from build123d import *

# Parameters (mm, degrees)
SKETCH_1_W               = 65
SKETCH_1_H               = 70
EXTRUDE_1_DEPTH          = 25
SKETCH_2_R               = 15.75
CUT_EXTRUDE_1_DEPTH      = 26
SKETCH_4_R               = 3
CUT_EXTRUDE_2_DEPTH      = 40
PATTERN_CIRCULAR_1_COUNT = 4
CUT_EXTRUDE_3_DEPTH      = 26
CUT_EXTRUDE_START        = -26
CUT_EXTRUDE_5_DEPTH      = 46
SKETCH_8_R               = 1.25
SKETCH_8_R_2             = 1.5
CUT_EXTRUDE_6_DEPTH      = 10
SKETCH_9_W               = 81.802440552
SKETCH_9_H               = 62.233215756
CUT_EXTRUDE_7_DEPTH      = 10


with BuildPart() as part:
    # 草图1 → 凸台-拉伸1 (new body)
    with BuildSketch(Plane.XY):
        with Locations((-15.56280925, 45.394966444)):
            Rectangle(SKETCH_1_W, SKETCH_1_H)
    extrude(amount=EXTRUDE_1_DEPTH)

    # 草图2 → 切除-拉伸1 (cut, through all)
    with BuildSketch(Plane.XY.offset(25)):
        with Locations((-15.56280925, 45.394966444)):
            Circle(SKETCH_2_R)
    extrude(amount=-CUT_EXTRUDE_1_DEPTH, mode=Mode.SUBTRACT)

    # 草图4 → 切除-拉伸2 (cut)
    with BuildSketch(Plane(origin=(0, 0, 0), x_dir=(-1, 0, 0), z_dir=(0, 0, -1))):
        with Locations((-7.18719075, 45.394966444)):
            Circle(SKETCH_4_R)
    cut_extrude_2 = extrude(amount=-CUT_EXTRUDE_2_DEPTH, mode=Mode.SUBTRACT)

    # 阵列(圆周)1: 切除-拉伸2 ×4 about axis
    pattern_circular_1_axis = Axis((-15.56280925, 45.394966444, 0), (0, 0, 1))
    for i in range(1, PATTERN_CIRCULAR_1_COUNT):
        add(cut_extrude_2.rotate(pattern_circular_1_axis, i * 360 / PATTERN_CIRCULAR_1_COUNT), mode=Mode.SUBTRACT)

    # 草图6 → 切除-拉伸3 (cut, through all)
    with BuildSketch(Plane.XY.offset(25)):
        with BuildLine():
            Line((-31.31280925, 45.394966444), (0.18719075, 45.394966444))
            ThreePointArc((0.18719075, 45.394966444), (8.56219075, 53.769966444), (16.93719075, 45.394966444))
            Line((16.93719075, 45.394966444), (16.93719075, 80.394966444))
            Line((16.93719075, 80.394966444), (-48.06280925, 80.394966444))
            Line((-48.06280925, 80.394966444), (-48.06280925, 45.394966444))
            ThreePointArc((-48.06280925, 45.394966444), (-39.68780925, 53.769966444), (-31.31280925, 45.394966444))
        make_face()
    extrude(amount=-CUT_EXTRUDE_3_DEPTH, mode=Mode.SUBTRACT)

    # 草图7 → 切除-拉伸5 (cut)
    with BuildSketch(Plane.XY.offset(25).offset(CUT_EXTRUDE_START)):
        with BuildLine():
            Line((-48.06280925, 45.394966444), (-48.06280925, 14.278358566))
            Line((-48.06280925, 14.278358566), (-42.197147473, 14.278358566))
            ThreePointArc((-42.197147473, 14.278358566), (-30.908342931, 25.972564608), (-42.993400823, 36.841922394))
            ThreePointArc((-42.993400823, 36.841922394), (-46.700248306, 40.423712469), (-48.06280925, 45.394966444))
        make_face()
    cut_extrude_5 = extrude(amount=CUT_EXTRUDE_5_DEPTH, mode=Mode.SUBTRACT)

    # 镜向1: 切除-拉伸5 across plane
    add(cut_extrude_5.mirror(Plane.ZY.offset(15.56280925)), mode=Mode.SUBTRACT)

    # 草图8 → 切除-拉伸6 (cut)
    with BuildSketch(Plane.XZ.offset(-10.394966444)):
        with Locations((-28.06280925, 12.5)):
            Circle(SKETCH_8_R)
        with Locations((-42.993400823, 12.5)):
            Circle(SKETCH_8_R_2)
        with Locations((-35.56280925, 6.25)):
            Circle(SKETCH_8_R_2)
    cut_extrude_6 = extrude(amount=-CUT_EXTRUDE_6_DEPTH, mode=Mode.SUBTRACT)

    # 镜向2: 切除-拉伸6 across plane
    add(cut_extrude_6.mirror(Plane.ZY.offset(15.56280925)), mode=Mode.SUBTRACT)

    # 草图9 → 切除-拉伸7 (cut)
    with BuildSketch(Plane(origin=(0, 0, 0), x_dir=(-1, 0, 0), z_dir=(0, 0, -1))):
        with Locations((15.56280925, 45.394966444)):
            Rectangle(SKETCH_9_W, SKETCH_9_H)
    extrude(amount=-CUT_EXTRUDE_7_DEPTH, mode=Mode.SUBTRACT)


solid = part.part
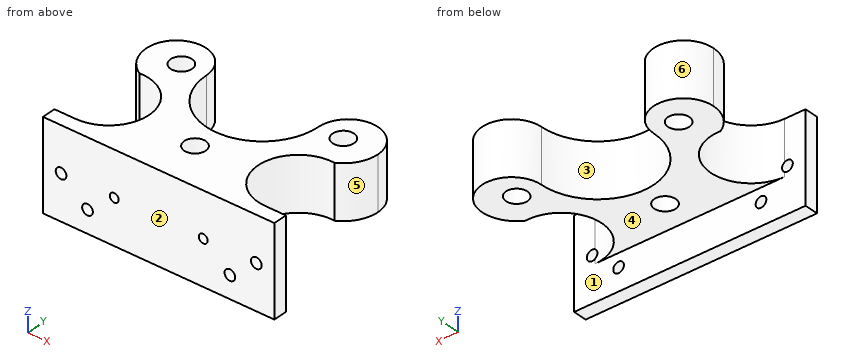
Check sheet for the modelled part. Datum: model origin and axes. Units: mm. Face numbers are marked on the shaded views. A direction names the side the tool comes from. Round coordinates to 2 decimals unless told otherwise and drop trailing zeros. Loops run counter-clockwise (first coordinate to the right, second up) from the corner with the lowest first, then second, coordinate; pieces in that order, holes last.
1. Mould release check, pull along Y, two halves, no side actions. Record for the marked faces 1, 2, 3 and 4: released by +Y, released by -Y, zero draft, split by the parting line, or undercut.
2. Sectioned sample at D-D on z = 12.5. Give the number of separate pieces and of enclosed holes in the cut face, and give its area (3 significant figures).
3. Gauge pin test, flat ends, axial feed: pin 1 Ø2.5 at (x, z) = (-42.99, 12.5) entering from +Y; pin 2 Ø7 at (x, y) = (-15.56, 22.64) entering from -Z; pin 3 Ø2.5 at (x, z) = (-35.56, 6.25) entering from -Y; pin 4 Ø2 at (x, z) = (-28.06, 12.5) entering from -Y. Record the tip position at first contact, or that the pin passes through.
4. Sectioned sample at A-A on z = 6.25. Record the boundary of the cut face in (x, y), and give its area (3 significant figures).
5. Sectioned sample at C-C on y = 31. Record the boundary of the cut face in (x, z), and give its area (3 significant figures).
6. Scan lines: probe 1 along Y at (x, z) = (7.5, 22.25); probe 2 along Y at (x, z) = (-36, 19); probe 3 along Y at (x, z) = (-31, 3). Record each from-to range of solid material in increasing order.
7. Sectioned sample at B-B on x = -16.5. Record the boundary of the cut face in (y, z), and give its area (3 significant figures).
8. Set-up check for the marked faces 5 and 6: record each of +Z, -Z, +X, -X, +Y, -Y from which the full face is reachable in a straight line by a thin tool's end or side.
Recorded:
1. face 1: undercut
1. face 2: released by -Y
1. face 3: released by +Y
1. face 4: zero draft
2. separate pieces: 3
2. enclosed holes: 3
2. area: 1,260 mm2
3. pin 1: stops at y = 53.51
3. pin 2: stops at z = 10
3. pin 3: passes through
3. pin 4: stops at y = 20.39
4. outline: (-48.06, 10.39) - (-37.06, 10.39) - (-37.06, 14.28) - (-48.06, 14.28) - close; (-34.06, 10.39) - (2.94, 10.39) - (2.94, 14.28) - (-34.06, 14.28) - close; (5.94, 10.39) - (16.94, 10.39) - (16.94, 14.28) - (5.94, 14.28) - close
4. area: 229 mm2
5. outline: (-32.29, 10) - (-21.95, 10) - (-21.95, 25) - (-32.29, 25) - close; (-9.17, 10) - (1.16, 10) - (1.16, 25) - (-9.17, 25) - close
5. area: 310 mm2
6. probe 1: y = 10.39 to 14.86, 36.29 to 42.41, 48.38 to 53.7
6. probe 2: y = 10.39 to 16.13, 35.02 to 43.48, 47.31 to 52.91
6. probe 3: y = 10.39 to 14.28
7. outline: (10.39, 0) - (14.28, 0) - (14.28, 10) - (19.8, 10) - (19.8, 25) - (10.39, 25) - close; (25.49, 10) - (29.67, 10) - (29.67, 25) - (25.49, 25) - close
7. area: 243 mm2
8. face 5: +Z, -Z, +X
8. face 6: +Z, -Z, +Y
